For this review, take the finished solid that the model builds, in its own axes (mm). Face numbers are marked on the shaded views. Coordinates: 2 decimals unless noted, no trailing zeros. Loops run counter-clockwise (first coordinate to the right, second up) from the corner with the lowest first, then second, coordinate; pieces in that order, holes last.
```python
from build123d import *

# Parameters (mm, degrees)
SKETCH2_R           = 60.49
SKETCH2_R_2         = 54.14
BOSS_EXTRUDE1_DEPTH = 876.3
SKETCH3_R           = 9.525
CUT_EXTRUDE1_DEPTH  = 438.15


with BuildPart() as part:
    # Sketch2 → Boss-Extrude1 (new body)
    with BuildSketch(Plane(origin=(0, 0, 0), x_dir=(1, 0, 0), z_dir=(0, 1, 0))):
        with Locations(Location((0, 0, 0), (0, 0, 270))):
            Circle(SKETCH2_R)
        with Locations(Location((0, 0, 0), (0, 0, 270))):
            Circle(SKETCH2_R_2, mode=Mode.SUBTRACT)
    extrude(amount=BOSS_EXTRUDE1_DEPTH)

    # Sketch3 → Cut-Extrude1 (cut, symmetric)
    with BuildSketch(Plane(origin=(0, 0, 0), x_dir=(0, 0, -1), z_dir=(1, 0, 0))):
        with Locations((0, 101.6)):
            Circle(SKETCH3_R)
        with Locations((0, 774.7)):
            Circle(SKETCH3_R)
    extrude(amount=CUT_EXTRUDE1_DEPTH, both=True, mode=Mode.SUBTRACT)


solid = part.part
```
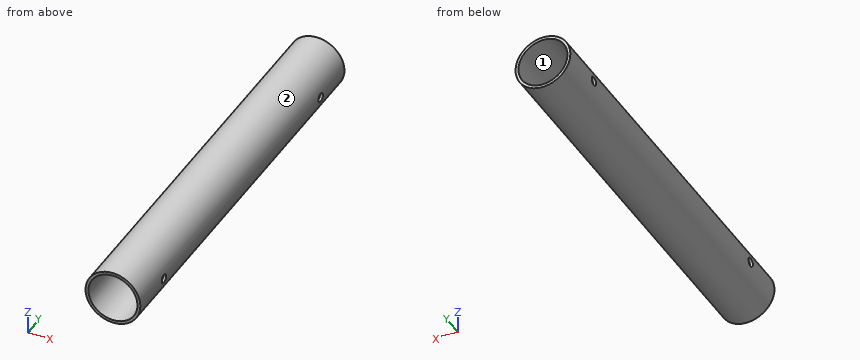
Q1. Consider section C-C (y = 796.5). State the section outline as (x, z) points, then the cut area to 3 significant figures.
Q2. Consider section B-B (z = 0). State the section outline as (x, y) points (3 decimals).
Q3. Wall thickness on probe 1 along Y at (x, z) = (55.25, 0) (3 decimals); probe 2 along X at (y, z) = (346, 0); probe 3 along X at (y, z) = (518.5, -4): over which ranges is each line inside the solid? List them lowest first.
Q4. The part is to be moulded in two halves that separate along X. For the marked faces 1 and 2, say which applies: +X half, -X half, draft (parallel to the pull), parting line (faces both ways), or undercut.
Q5. For pin 1 Ø6 at (y, z) = (458, -32) entering from +X; pin 2 Ø10 at (y, z) = (370.5, 18.5) entering from +X; pin 3 Ø1.5 at (y, z) = (239.5, -27) entering from -X, all flat-tipped, find the tip position at first contact; note any pin that passes through.
Q6. Consider section D-D (z = -46). State the section outline as (x, y) points, then the cut area to 3 significant figures.
Q7. Consider section A-A (x = 0). State the section outline as (y, z) points.
Model answer:
1. outline: circle Ø120.98 at (0, 0); hole circle Ø108.28 at (0, 0)
1. area: 2,290 mm2
2. outline: (-60.49, 0) - (-54.14, 0) - (-54.14, 92.075) - (-60.49, 92.075) - close; (-60.49, 111.125) - (-54.14, 111.125) - (-54.14, 765.175) - (-60.49, 765.175) - close; (-60.49, 784.225) - (-54.14, 784.225) - (-54.14, 876.3) - (-60.49, 876.3) - close; (54.14, 0) - (60.49, 0) - (60.49, 92.075) - (54.14, 92.075) - close; (54.14, 111.125) - (60.49, 111.125) - (60.49, 765.175) - (54.14, 765.175) - close; (54.14, 784.225) - (60.49, 784.225) - (60.49, 876.3) - (54.14, 876.3) - close
3. probe 1: y = 0 to 92.075, 111.125 to 765.175, 784.225 to 876.3
3. probe 2: x = -60.49 to -54.14, 54.14 to 60.49
3. probe 3: x = -60.36 to -53.99, 53.99 to 60.36
4. face 1: undercut
4. face 2: parting line
5. pin 1: stops at x = 53.09
5. pin 2: stops at x = 58.96
5. pin 3: stops at x = -54.5
6. outline: (-39.28, 0) - (-28.55, 0) - (-28.55, 876.3) - (-39.28, 876.3) - close; (28.55, 0) - (39.28, 0) - (39.28, 876.3) - (28.55, 876.3) - close
6. area: 18,800 mm2
7. outline: (0, -60.49) - (876.3, -60.49) - (876.3, -54.14) - (0, -54.14) - close; (0, 54.14) - (876.3, 54.14) - (876.3, 60.49) - (0, 60.49) - close
